Model file for the job. Use its own axes, mm. Coordinates: 2 decimals unless noted, no trailing zeros. Order: outer loops, then holes, each group sorted by start corner. A loop starts at its lowest first (then second) coordinate and runs counter-clockwise, first axis right, second up. Notation, with made-up numbers: (22, 18.5) -> (78, 18.5) arc R30 cw to (78, 56.5) -> close; hole circle Ø7 at (-10, 21.25). An arc over 180 degrees is marked (long way). Use CSV: the item, a comma, the result in double quotes. Start each with the question number.
(1) Cut at B-B on y = -75. Write the cut outline in (x, z), plus the area to 3 significant figures.
(2) Cut at A-A on z = -5.25. Write the cut outline in (x, y), plus the area to 3 significant figures.
(3) Cut at C-C on x = -95. Write the cut outline in (y, z), plus the area to 3 significant figures.
(4) Probe L1, parallel to Z at x = -43, y = -28; L2, parallel to X at y = -79, z = 9.5; L3, parallel to Y at x = -46, z = 5. List the from-to ranges inside material, lowest first.
(5) Cut at D-D on y = -18. Write the cut outline in (x, z), plus the area to 3 significant figures.
(6) Pin check, flat tips, straight feed: pin 1 Ø17 at (x, y) = (-95, -75) entering from +Z; pin 2 Ø5 at (y, z) = (-14, -3.5) entering from -X; pin 3 Ø5 at (x, z) = (-1, 14) entering from +Y; pin 4 Ø8 at (x, y) = (-115.5, -11.5) entering from -Z. Stop position of each tip, or through.
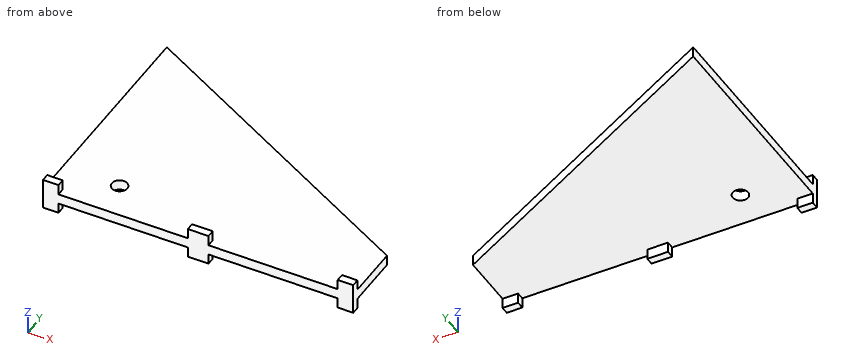
```python
from build123d import *

# Parameters (mm, degrees)
F0_R     = 7.5
F1_DEPTH = 10
F2_W     = 15
F2_H     = 7.5
F2_W_2   = 20
F3_DEPTH = 10
F4_W     = 15
F4_H     = 7.5
F4_W_2   = 20
F5_DEPTH = 10


with BuildPart() as f1:
    # F0 (on Top) → F1 (new body)
    with BuildSketch(Plane.XY):
        Polygon((150, -50), (-150, 110), (-150, -110), (150, -110), align=None)
        with Locations((-95, -75)):
            Circle(F0_R, mode=Mode.SUBTRACT)
    extrude(amount=F1_DEPTH)

    # F2 (on face) → F3 (join)
    with BuildSketch(Plane.XY.offset(10)):
        with Locations((-142.5, -106.25)):
            Rectangle(F2_W, F2_H)
        with Locations((142.5, -106.25)):
            Rectangle(F2_W, F2_H)
        with Locations((0, -106.25)):
            Rectangle(F2_W_2, F2_H)
    extrude(amount=F3_DEPTH)

    # F4 (on face) → F5 (join)
    with BuildSketch(Plane(origin=(0, 0, 0), x_dir=(1, 0, 0), z_dir=(0, 0, -1))):
        with Locations((-142.5, 106.25)):
            Rectangle(F4_W, F4_H)
        with Locations((142.5, 106.25)):
            Rectangle(F4_W, F4_H)
        with Locations((0, 106.25)):
            Rectangle(F4_W_2, F4_H)
    extrude(amount=F5_DEPTH)


solid = f1.part
```
Outcome:
1,outline,"(-150, 0) -> (-102.5, 0) -> (-102.5, 10) -> (-150, 10) -> close; (-87.5, 0) -> (150, 0) -> (150, 10) -> (-87.5, 10) -> close"
1,area,"2,850 mm2"
2,outline,"(-150, -110) -> (-135, -110) -> (-135, -102.5) -> (-150, -102.5) -> close; (-10, -110) -> (10, -110) -> (10, -102.5) -> (-10, -102.5) -> close; (135, -110) -> (150, -110) -> (150, -102.5) -> (135, -102.5) -> close"
2,area,"375 mm2"
3,outline,"(-110, 0) -> (-82.5, 0) -> (-82.5, 10) -> (-110, 10) -> close; (-67.5, 0) -> (80.67, 0) -> (80.67, 10) -> (-67.5, 10) -> close"
3,area,"1,760 mm2"
4,L1,"0 to 10"
4,L2,"-150 to -101.34, -88.66 to 150"
4,L3,"-110 to 54.53"
5,outline,"(-150, 0) -> (90, 0) -> (90, 10) -> (-150, 10) -> close"
5,area,"2,400 mm2"
6,pin 1,"z = 10"
6,pin 2,"through"
6,pin 3,"y = -102.5"
6,pin 4,"z = 0"
